```python
from build123d import *

# Parameters (mm, degrees)
SKETCH2_R          = 2.1
CUT_EXTRUDE1_DEPTH = 54.600373133
FILLET1_R          = 2


with BuildPart() as part:
    # Sketch1 → Revolve1 (revolve)
    with BuildSketch(Plane.XY, mode=Mode.PRIVATE) as revolve1_sk:
        Polygon((-70.7, 11), (-68.7, 11), (-68.7, 12), (-67.7, 12), (-67.7, 11), (-60.7, 11), (-60.7, 9), (-41.7, 9), (-41.7, 11), (-34.7, 11), (-34.7, 12), (-33.7, 12), (-33.7, 11.038518603), (-31.7, 11.038518603), (-31.7, 26), (-38.7, 26), (-38.7, 16), (-70.7, 16), align=None)
    revolve(revolve1_sk.sketch.rotate(Axis((-70.7, 0, 0), (1, 0, 0)), 180), axis=Axis((-70.7, 0, 0), (1, 0, 0)))

    # Sketch2 → Cut-Extrude1 (cut, through all)
    with BuildSketch(Plane(origin=(-31.7, 0, 0), x_dir=(0, 0, -1), z_dir=(1, 0, 0))):
        with Locations((0, 21)):
            Circle(SKETCH2_R)
        with Locations((21, 0)):
            Circle(SKETCH2_R)
        with Locations((0, -21)):
            Circle(SKETCH2_R)
        with Locations((-21, 0)):
            Circle(SKETCH2_R)
    extrude(amount=-CUT_EXTRUDE1_DEPTH, mode=Mode.SUBTRACT)

    # Fillet1
    fillet1_edges = [part.edges().sort_by_distance(p)[0] for p in [
        (-70.7, 16, 0),
        (-31.7, 26, 0),
    ]]
    fillet(fillet1_edges, radius=FILLET1_R)


solid = part.part
```
Geometry: final body of the model. Coordinates: model frame, mm. A direction names the side the tool comes from. Round coordinates to 2 decimals unless told otherwise and drop trailing zeros. Write each loop counter-clockwise with the first axis right and the second up, starting at its lowest first coordinate (ties: lowest second). Pieces come first, ordered by that corner, then holes. Notation, with made-up numbers: (8.5, -37.75) -> (51.5, -37.75) arc R23 cw to (51.5, -1.75) -> close; hole circle Ø6 at (-26, 69). An arc over 180 degrees is marked (long way). Return JSON: item names as keys, results as strings.
Q1. Section B-B on y = 0. Give the number of separate pieces and of enclosed holes in the cut face, and give its area (3 significant figures).
From the geometry:
{"separate pieces": "4", "enclosed holes": "0", "area": "540 mm2"}
Q2. Mould query, pull axis Z, two halves, no side actions, for faces 1 (the flat face through (-31.7, 10.3, 5)), 2 (the flat face through (-41.7, 2, 9)), 3 (the cylindrical face through (-53.91, 3.47, 15.62)), 4 (the flat face through (-34.7, 5, 10)). Classes: +Z half, -Z half, draft (parallel to the pull), parting line (faces both ways), or undercut.
From the geometry:
{"face 1": "draft", "face 2": "undercut", "face 3": "parting line", "face 4": "undercut"}
Q3. Section A-A on x = -36. Return the cut outline in (y, z).
From the geometry:
{"outline": "circle Ø52 at (0, 0); hole circle Ø4.2 at (-21, 0); hole circle Ø22 at (0, 0); hole circle Ø4.2 at (0, -21); hole circle Ø4.2 at (0, 21); hole circle Ø4.2 at (21, 0)"}
Q4. Ray query, line 1 (X direction, y = 12, z = 21); line 2 (Y direction, x = -44, z = 5); line 3 (Z direction, x = -46, y = -8). Return the intervals inside material, ascending.
From the geometry:
{"line 1": "-38.7 to -31.71", "line 2": "-15.2 to -7.48, 7.48 to 15.2", "line 3": "-13.86 to -4.12, 4.12 to 13.86"}
Q5. Section D-D on x = -67. Return the cut outline in (y, z).
From the geometry:
{"outline": "circle Ø32 at (0, 0); hole circle Ø22 at (0, 0)"}
Q6. First-contact query: pin 1 Ø4 at (x, z) = (-39.5, 11) entering from +Y; pin 2 Ø8 at (x, z) = (-41.5, 17) entering from +Y; pin 3 Ø4 at (y, z) = (8, 4) entering from +X. Flat tips, straight axial feed; report the tip coordinate or a pass-through.
From the geometry:
{"pin 1": "y = 24.33", "pin 2": "y = 21.82", "pin 3": "x = -41.7"}
Q7. Set-up query: faces 5 (the cylindrical face through (-34.193, -11.446, -3.604)), 6 (the flat face through (-60.7, -2, 9)), 7 (the cylindrical face through (-38.15, 2.38, 10.74)), 8 (the cylindrical face through (-35.151, 0.631, 18.997)). Return all of +Z, -Z, +X, -X, +Y, -Y with unobstructed straight access to the full face (end or side cutting, diameter ignored); none if empty.
From the geometry:
{"face 5": "none", "face 6": "-X", "face 7": "+X", "face 8": "+X, -X"}
